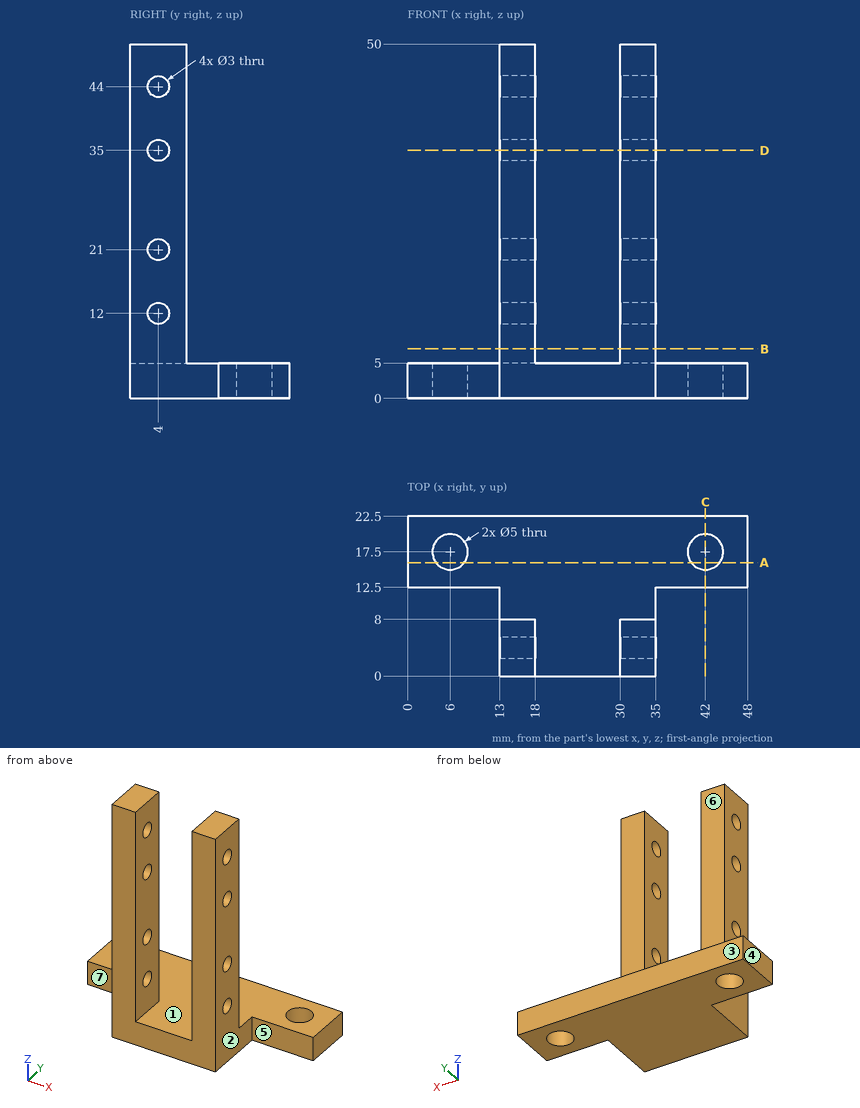
Can you work these out from the drawing? Everything is in mm from the part's minimum corner. A direction names the side the tool comes from. Give positions to 0.01 mm unless a question says otherwise; leave off trailing zeros. Order: outer loops, then holes, each group sorted by start corner. A loop starts at its lowest first (then second) coordinate and runs counter-clockwise, first axis right, second up. Notation, with made-up numbers: M 61,-19.75 L 105,-19.75 A10 ccw 105,-6.75 Z; hole C -37,-39.5 d6. An arc over 180 degrees is marked long. Use a Markdown table: item, result. Add a question column.
1. Suppose I cut it at B-B (z = 7). List the corners of the cut face in (x, y) for me.
2. For pin 1 Ø3.5 at (y, z) = (4, 44) entering from +X; pin 2 Ø4 at (x, z) = (20.5, 29) entering from +Y; pin 3 Ø4 at (y, z) = (4, 12) entering from -X; pin 4 Ø6 at (x, z) = (11.5, 41.5) entering from +Y, each with a flat end and sliding along its axis, tell me the tip position at first contact or that it passes through.
3. On a 3-axis mill with a long thin cutter (end or side, diameter ignored), from which of +Z, -Z, +X, -X, +Y, -Y can I reach the whole of each face in a straight line? I mean the marked faces 5, 6 and 7. Say none if no direction works.
4. If we mould it in two halves opening along X, with no side actions, what happens to the marked faces 1, 2, 3 and 4? For each: +X half, -X half, draft (parallel to the pull), parting line (faces both ways), or undercut.
5. Suppose I cut it at C-C (x = 42). List the corners of the cut face in (y, z) for me, and give its area (3 significant figures).
6. Suppose I cut it at A-A (y = 16). List the corners of the cut face in (x, z) for me.
7. Suppose I cut it at D-D (z = 35). List the corners of the cut face in (x, y) for me.
8. I need wall thicknesses on probe 1 along Z at (x, y) = (33.35, 4); probe 2 along X at (y, z) = (2.5, 35.5); probe 3 along Y at (x, z) = (42, 3.2). Which ranges of each line are inside material? Lowest first, please. Write a range as from..to.
Results list:
| question | item | result |
|---|---|---|
| 1 | outline | M 13,0 L 18,0 L 18,8 L 13,8 Z; M 30,0 L 35,0 L 35,8 L 30,8 Z |
| 2 | pin 1 | stops at x = 35 |
| 2 | pin 2 | passes through |
| 2 | pin 3 | stops at x = 13 |
| 2 | pin 4 | stops at y = 8 |
| 3 | face 5 | +Z, -Z, +X, -Y |
| 3 | face 6 | +Z, +X, -X, +Y |
| 3 | face 7 | +Z, -Z, -X, -Y |
| 4 | face 1 | undercut |
| 4 | face 2 | +X half |
| 4 | face 3 | draft |
| 4 | face 4 | -X half |
| 5 | outline | M 12.5,0 L 15,0 L 15,5 L 12.5,5 Z; M 20,0 L 22.5,0 L 22.5,5 L 20,5 Z |
| 5 | area | 25.0 mm² |
| 6 | outline | M 0,0 L 4,0 L 4,5 L 0,5 Z; M 8,0 L 40,0 L 40,5 L 8,5 Z; M 44,0 L 48,0 L 48,5 L 44,5 Z |
| 7 | outline | M 13,0 L 18,0 L 18,2.5 L 13,2.5 Z; M 13,5.5 L 18,5.5 L 18,8 L 13,8 Z; M 30,0 L 35,0 L 35,2.5 L 30,2.5 Z; M 30,5.5 L 35,5.5 L 35,8 L 30,8 Z |
| 8 | probe 1 | z = 0..10.5, 13.5..19.5, 22.5..33.5, 36.5..42.5, 45.5..50 |
| 8 | probe 2 | x = 13..18, 30..35 |
| 8 | probe 3 | y = 12.5..15, 20..22.5 |
